Read the model definition and answer for the solid it produces. Units are mm, in the model's axes. A direction names the side the tool comes from. Coordinates: 2 decimals unless noted, no trailing zeros. Order: outer loops, then holes, each group sorted by start corner. A loop starts at its lowest first (then second) coordinate and runs counter-clockwise, first axis right, second up.
Autodesk Inventor part; units mm, degrees
ref_plane "YZ Plane" through (0, 0, 0) normal (1, 0, 0) x (0, 1, 0)
ref_plane "XZ Plane" through (0, 0, 0) normal (0, 1, 0) x (-1, 0, 0)
ref_plane "XY Plane" through (0, 0, 0) normal (0, 0, 1) x (1, 0, 0)
sketch "Sketch1" plane through (0, 0, 0) normal (0, 1, 0) x (-1, 0, 0)
  line L0 (0, 0) -> (0, 150.5)
  line L1 (47.6822, -16.05) -> (47.6822, -184.7082) construction
  line L2 (47.6822, -184.7082) -> (-45.5409, -184.7082) construction
  line L3 (-45.5409, -184.7082) -> (-45.5409, -16.05) construction
  line L4 (-45.5409, -16.05) -> (47.6822, -16.05) construction
  line L5 (51, 71) -> (51, 72) construction
  line L6 (53, 71) -> (53, 72) construction
  line L7 (49, 72) -> (49, 71) construction
  arc A0 (49, 71) -> (53, 71) centre (51, 71) ccw construction
  arc A1 (53, 72) -> (49, 72) centre (51, 72) ccw construction
  line L8 (0, 85) -> (64.5191, 85) construction
  line L9 (51, 99) -> (51, 98) construction
  line L10 (53, 99) -> (53, 98) construction
  line L11 (49, 98) -> (49, 99) construction
  arc A2 (53, 99) -> (49, 99) centre (51, 99) ccw construction
  arc A3 (49, 98) -> (53, 98) centre (51, 98) ccw construction
  line L12 (50, 115) -> (-55, 115)
  line L13 (-55, 115) -> (-55, 55) construction
  line L14 (-55, 55) -> (50, 55)
  line L15 (55, 60) -> (55, 110)
  circle A4 centre (50, 60) radius 1.6
  circle A5 centre (51, 71.5) radius 2
  circle A6 centre (51, 98.5) radius 2
  line L16 (0, 57.5) -> (37.5, 57.5)
  line L17 (42.5, 62.5) -> (42.5, 107.5)
  line L18 (37.5, 112.5) -> (0, 112.5)
  circle A7 centre (50, 110) radius 1.6
  line L19 (50, 60) -> (50, 110) construction
  arc A8 (50, 55) -> (55, 60) centre (50, 60) ccw
  arc A9 (55, 110) -> (50, 115) centre (50, 110) ccw
  arc A10 (37.5, 57.5) -> (42.5, 62.5) centre (37.5, 62.5) ccw
  arc A11 (42.5, 107.5) -> (37.5, 112.5) centre (37.5, 107.5) ccw
  point P0 (51, 74)
  point P1 (51, 69)
  point P2 (51, 96)
  point P3 (51, 101)
  point P4 (55, 115)
  point P5 (55, 55)
  point P6 (0, 55)
  point P7 (0, 115)
  point P8 (42.5, 57.5)
  point P9 (42.5, 112.5)
  point P10 (0, 113)
  dimension "d9" = 4
  dimension "d10" = 5
  dimension "d12" = 51
  dimension "d22" = 27
  dimension "d29" = 110
  dimension "d31" = 55
  dimension "d85" = 2.5
  dimension "d86" = 42.5
  dimension "d91" = 3.2
  dimension "d92" = 50
  dimension "d99" = 5
extrude "Extrusion1" add sketch "Sketch1" along normal blind 5 contours L16 A10 L17 A11 L18 L0 L12 A9 L15 A8 L14
sketch "Sketch4" plane through (0, 5, 0) normal (0, 1, 0) x (1, 0, 0)
  circle A0 centre (-50, -60) radius 1.6 construction
  circle A1 centre (-50, -60) radius 3
  circle A2 centre (-50, -110) radius 1.6 construction
  circle A3 centre (-50, -110) radius 3
  point P0 (0, 0)
  dimension "d93" = 6
extrude "Extrusion5" cut sketch "Sketch4" against normal blind 2.5
sketch "Sketch7" plane through (0, 0, 115) normal (1, 0, 0) x (0, 0, -1)
  line L0 (0, 0) -> (2.5, 0) construction
  line L1 (2.5, 0) -> (2.5, 5) construction
  line L2 (0, 5) -> (2.5, 5) construction
  line L3 (0, 0) -> (0, 5)
  line L4 (2.5, 0) -> (-25.7843, 0)
  line L5 (-25.7843, 0) -> (2.5, 28.2843)
  line L6 (2.5, 28.2843) -> (2.5, 0)
  line L7 (2.5, 0) -> (2.5, 5)
  line L8 (-22.2487, 0) -> (2.5, 24.7487)
  line L9 (0, 5) -> (0, 22.2487)
  line L10 (-23.2843, 2.5) -> (2.5, 2.5)
  line L11 (2.5, 24.7487) -> (0.7322, 26.5165)
  arc A0 (2.5, 24.7487) -> (0.7322, 26.5165) centre (1.6161, 25.6326) ccw
  arc A1 (-17.2487, 8.5355) -> (-13.7132, 0) centre (-13.7132, 5) ccw
  arc A2 (-15.481, 6.7678) -> (-13.7132, 2.5) centre (-13.7132, 5) ccw
  line L12 (-11.6421, 14.1421) -> (-17.2639, 19.7639) construction
  arc A3 (-2.5, 2.5) -> (0, 5) centre (-2.5, 5) ccw
  line L13 (0, 0) -> (0, 5)
  point P0 (115, 0)
  point P1 (-19.7487, 2.5)
  point P2 (0, 2.5)
  dimension "d159" = 2.5
  dimension "d160" = 45
  dimension "d161" = 40
  dimension "d184" = 2.5
  dimension "d197" = 5
extrude "Extrusion15" add sketch "Sketch7" against normal blind 20 contours L4 A1 L10 L3 | L3 L10 L6 L4 | L10 A3 L3 | A1 L8 A2 L10 | L8 A1 L5 L11 | L11 A0 L6 | L6 A0
sketch "Sketch9" plane through (-20, 28.2843, 112.5) normal (0, 0.7071, 0.7071) x (1, 0, 0)
  circle A0 centre (10, -10) radius 2.5
  line L0 (20, -2.5) -> (20, -27.9289) construction
  line L1 (0, -27.9289) -> (0, -2.5) construction
  line L2 (0, -15) -> (20, -15) construction
  circle A1 centre (10, -20) radius 2.5
  line L3 (20, -27.9289) -> (0, -27.9289) construction
  circle A2 centre (10, -10) radius 4.5
  circle A3 centre (10, -10) radius 5 construction
  line L4 (10, -20) -> (10, -10) construction
  line L5 (10, -10) -> (20, -10) construction
  line L6 (10, -20) -> (20, -20) construction
  circle A4 centre (10, -20) radius 4.5
  circle A5 centre (10, -20) radius 5 construction
  line L7 (20, -2.5) -> (0, -2.5) construction
  line L8 (20, 0) -> (0, 0) construction
  point P0 (20, 59.5495)
  dimension "d183" = 5
  dimension "d187" = 9
  dimension "d188" = 10
  dimension "d189" = 10
  dimension "d195" = 2.5
  dimension "d196" = 15
  dimension "d198" = 10
extrude "Extrusion16" cut sketch "Sketch9" against normal up to next contours A0 | A1 | A2 | A4
extrude "Extrusion17" add sketch "Sketch9" against normal blind 1.25
mirror "Mirror2" about plane through (0, 0, 0) normal (1, 0, 0)
properties part number "pad"
1) Which of the six approach directions +Z, -Z, +X, -X, +Y, -Y give full straight-line access (tool end or side, diameter ignored) to faces 1 (the flat face through (11.937, 18.96, 120.057)), 2 (the cylindrical face through (52.21, 3.77, 62.03)), 3 (the flat face through (42.5, 2, 85))?
A:
face 1: none
face 2: +Y
face 3: +Y, -Y
2) Determine the mould class of faces 4 (the cylindrical face through (50.74, 2.465, 73.483)), 5 (the cylindrical face through (54, 2, 113)) for opening direction Z: pulls with the +Z half, pulls with the -Z half, needs draft (parallel to the pull), parting line crosses it, or undercut.
A:
face 4: undercut
face 5: pulls with the +Z half
3) A cutting plane is placed at B-B, the plane z = 98.5. Determine the outline of the cut face in (x, y), and give its area (3 significant figures).
A:
outline: (-55, 0) - (-53, 0) - (-53, 5) - (-55, 5) - close; (-49, 0) - (-42.5, 0) - (-42.5, 5) - (-49, 5) - close; (42.5, 0) - (49, 0) - (49, 5) - (42.5, 5) - close; (53, 0) - (55, 0) - (55, 5) - (53, 5) - close
area: 85.0 mm2
4) Straight lines are drawn through the part: line 1 (Z direction, x = 36, y = 2.5); line 2 (X direction, y = 1.45, z = 110); line 3 (Z direction, x = -51, y = 1.8). For each, find the intervals that lie inside material, in ascending order.
A:
line 1: z = 55 to 57.5, 112.5 to 115
line 2: x = -55 to -51.6, -48.4 to -41.83, 41.83 to 48.4, 51.6 to 55
line 3: z = 55.1 to 58.75, 61.25 to 69.5, 73.5 to 96.5, 100.5 to 108.75, 111.25 to 114.9
5) Flat-ended cylindrical pins translate along their axes: pin 1 Ø0.8 at (y, z) = (2, 126.5) entering from +X; pin 2 Ø9 at (x, z) = (-11.5, 125.5) entering from +Y; pin 3 Ø4 at (x, z) = (-50, 110) entering from +Y. Find the tip coordinate at first contact, or state that the pin passes through.
A:
pin 1: stops at x = 20
pin 2: stops at y = 19.78
pin 3: stops at y = 2.5
6) A cutting plane is placed at A-A, the plane x = -40.5. Determine the outline of the cut face in (y, z).
A:
outline: (0, 55) - (5, 55) - (5, 58.5) - (0, 58.5) - close; (0, 111.5) - (5, 111.5) - (5, 115) - (0, 115) - close
